Here's the drawing with two shaded views (mm, measured from the low corner). I have some questions. A direction names the side the tool comes from. Round coordinates to 2 decimals unless told otherwise and drop trailing zeros. Loops run counter-clockwise (first coordinate to the right, second up) from the corner with the lowest first, then second, coordinate; pieces in that order, holes last.
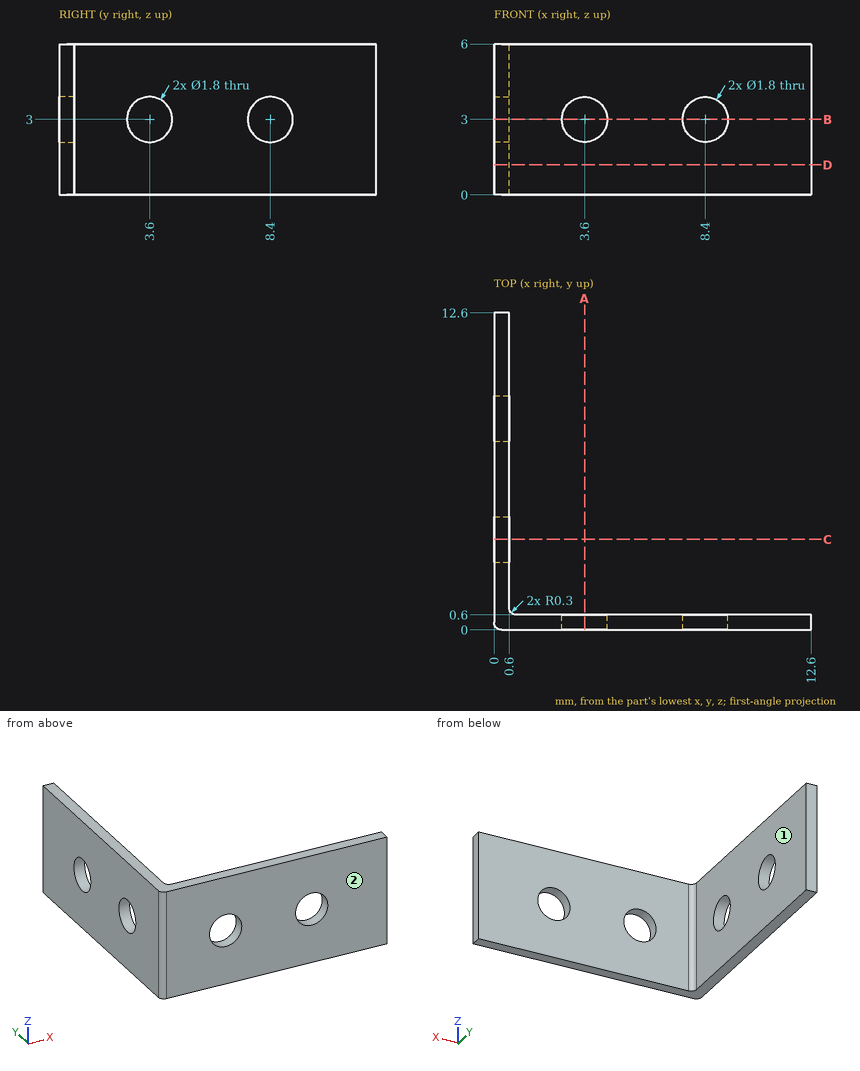
(1) If I drill on line 1 (X direction, y = 0.45, z = 3); line 2 (Y direction, x = 1.25, z = 0.6), over which ranges is the centre line in solid material (lowest first)?
Worked answers:
line 1: x = 0 to 2.7, 4.5 to 7.5, 9.3 to 12.6
line 2: y = 0 to 0.6
(2) If we section it at D-D, the plane z = 1.2: List the corners of the cut face in (x, y) for me.
Worked answers:
outline: (0, 0.3) arc R0.3 ccw to (0.3, 0) - (12.6, 0) - (12.6, 0.6) - (0.9, 0.6) arc R0.3 cw to (0.6, 0.9) - (0.6, 12.6) - (0, 12.6) - close
(3) If we section it at B-B, the plane z = 3: List the corners of the cut face in (x, y) for me, then the cut area to 3 significant figures.
Worked answers:
outline: (0, 0.3) arc R0.3 ccw to (0.3, 0) - (2.7, 0) - (2.7, 0.6) - (0.9, 0.6) arc R0.3 cw to (0.6, 0.9) - (0.6, 2.7) - (0, 2.7) - close; (0, 4.5) - (0.6, 4.5) - (0.6, 7.5) - (0, 7.5) - close; (0, 9.3) - (0.6, 9.3) - (0.6, 12.6) - (0, 12.6) - close; (4.5, 0) - (7.5, 0) - (7.5, 0.6) - (4.5, 0.6) - close; (9.3, 0) - (12.6, 0) - (12.6, 0.6) - (9.3, 0.6) - close
area: 10.4 mm2
(4) If we section it at A-A, the plane x = 3.6: List the corners of the cut face in (y, z) for me, then the cut area to 3 significant figures.
Worked answers:
outline: (0, 0) - (0.6, 0) - (0.6, 2.1) - (0, 2.1) - close; (0, 3.9) - (0.6, 3.9) - (0.6, 6) - (0, 6) - close
area: 2.52 mm2
(5) Will these pins go through, and if not, where does the flat tip stop? P1, Ø1.6, axis at x = 8.4, z = 3, coming from the -Y side; P2, Ø1.5, axis at x = 5, z = 0.5, coming from the +Y side; P3, Ø2, axis at y = 5, z = 3.5, coming from the +X side.
Worked answers:
P1: passes through
P2: stops at y = 0.6
P3: stops at x = 0.6
(6) For the marked faces 1 and 2, which set-ups out of +Z, -Z, +X, -X, +Y, -Y let a thin tool reach every point of the face, with its end or its side?
Worked answers:
face 1: +Z, -Z, +X, +Y
face 2: +Z, -Z, +X, -X, -Y
